The drawing under review shows one solid part. Ordinate dimensions are in mm from its lowest x, y, z. A direction names the side the tool comes from. Coordinates: 2 decimals unless noted, no trailing zeros. Order: outer loops, then holes, each group sorted by start corner. A loop starts at its lowest first (then second) coordinate and runs counter-clockwise, first axis right, second up.
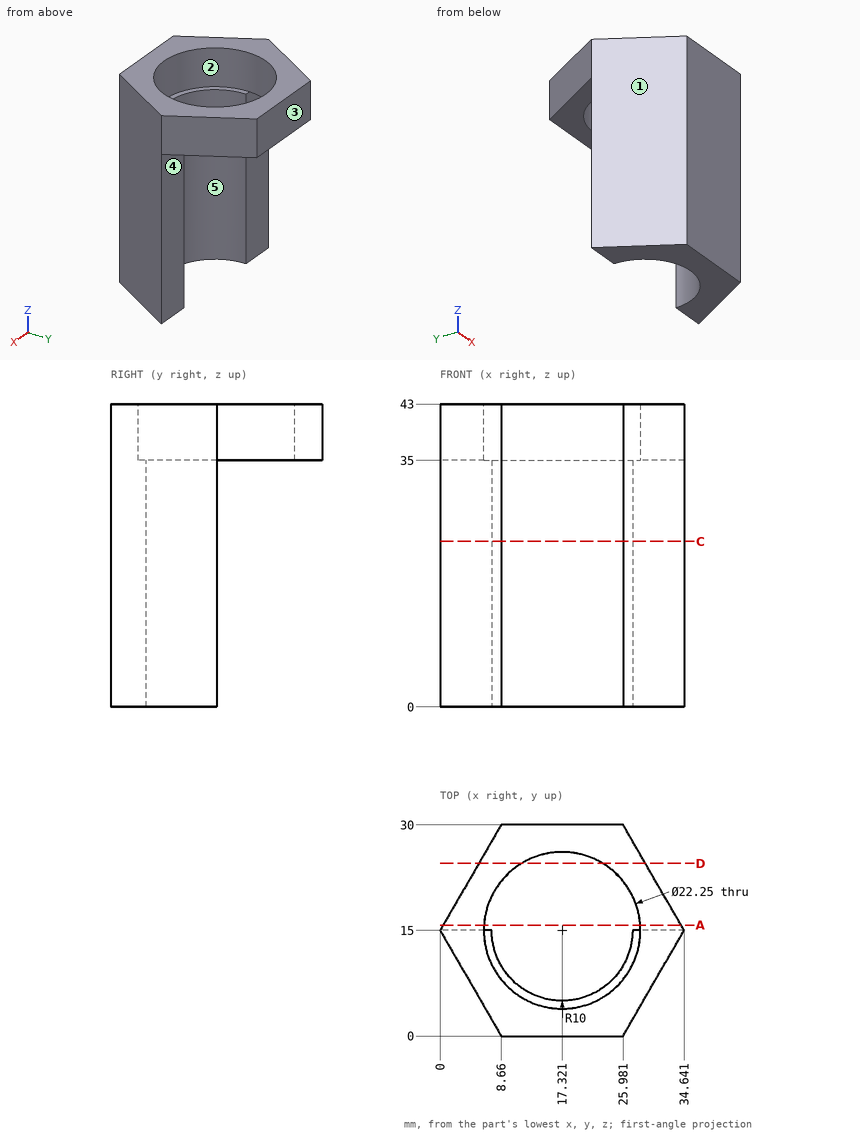
1. Add section A-A (y = 15.75). Give the boundary of the cut face in (x, z).
2. Add section D-D (y = 24.5). Give the boundary of the cut face in (x, z) (1 decimal).
3. To check wall thickness, follow line 1 (X direction, y = 15, z = 41.25) (1 decimal); line 2 (Z direction, x = 10.5, y = 7); line 3 (Z direction, x = 11, y = 27.5). State the ranges of each line that lie inside material, in increasing order.
4. Mouldability with a two-part tool opening along X and no side actions: class the marked faces 1, 2 and 3 as pulls with the +X half, pulls with the -X half, needs draft (parallel to the pull), parting line crosses it, or undercut.
5. Insertion check: pin 1 (16.5 mm diameter, centred on x = 23, y = 22.5, fed in from -Z); pin 2 (8 mm diameter, centred on x = 24.5, z = 17, fed in from +Y); pin 3 (3 mm diameter, centred on x = 24, y = 9.5, fed in from +Z); pin 4 (2 mm diameter, centred on x = 17.5, y = 8, fed in from +Z). Each pin has a flat end and moves straight along its axis. Give the tip position at first contact, or say it passes through.
6. For the marked faces 4 and 5, list the 3-axis set-ups (+Z, -Z, +X, -X, +Y, -Y) from which the entire face can be reached by the end or side of a thin tool; tool diameter is ignored.
7. Add section C-C (z = 23.5). Give the boundary of the cut face in (x, y), and give its area (3 significant figures).
Solution:
1. outline: (0.43, 35) - (6.22, 35) - (6.22, 43) - (0.43, 43) - close; (28.42, 35) - (34.21, 35) - (34.21, 43) - (28.42, 43) - close
2. outline: (5.5, 35) - (11.5, 35) - (11.5, 43) - (5.5, 43) - close; (23.1, 35) - (29.2, 35) - (29.2, 43) - (23.1, 43) - close
3. line 1: x = 0 to 6.2, 28.4 to 34.6
3. line 2: z = 0 to 35
3. line 3: z = 35 to 43
4. face 1: pulls with the -X half
4. face 2: undercut
4. face 3: needs draft
5. pin 1: stops at z = 35
5. pin 2: stops at y = 15
5. pin 3: stops at z = 35
5. pin 4: passes through
6. face 4: -Z, +X, -X, +Y
6. face 5: +Z, -Z, +Y
7. outline: (0, 15) - (8.66, 0) - (25.98, 0) - (34.64, 15) - (27.32, 15) arc R10 cw to (7.32, 15) - close
7. area: 233 mm2
